The listing builds one solid part. Answer for the finished solid, in the listing's coordinates (mm). A direction names the side the tool comes from. Coordinates: 2 decimals unless noted, no trailing zeros. Order: outer loops, then holes, each group sorted by start corner. A loop starts at its lowest first (then second) coordinate and runs counter-clockwise, first axis right, second up. Notation, with made-up numbers: M 74,-26 L 93,-26 A25 ccw 93,11 Z; hole C -16,89.5 d11. An arc over 180 degrees is marked long. One line per item, written item: value. Start each with the question number.
Q1. The part is cut by section C-C on z = 73. Give the vertices of the cut face in (x, y).
Q2. The part is cut by section A-A on y = -196. Give the vertices of the cut face in (x, z).
Q3. Straight lines are drawn through the part: line 1 along Y through (x, z) = (38.5, 49); line 2 along Z through (x, y) = (166.5, -106.5); line 3 along Z through (x, y) = (140, -156). For each, find the intervals that lie inside material, in ascending order. Write a range as [from, to].
Q4. The part is cut by section B-B on x = 130. Give the vertices of the cut face in (y, z), then the cut area to 3 significant figures.
Q5. For faces 1 (the flat face through (160, 0, 65)), 2 (the cylindrical face through (68.872, -33.32, 32.944)), determine the directions among +Z, -Z, +X, -X, +Y, -Y from which every point of the face is accessible in a straight line to the end or side of a thin tool.
Q6. The part is cut by section D-D on x = 160.5. Give the vertices of the cut face in (y, z), then the cut area to 3 significant figures.
Q7. Each of these flat-tipped pins is pushed along its axis until it touches: pin 1 Ø2 at (y, z) = (-89, 57) entering from -X; pin 2 Ø3 at (x, y) = (119.5, -97) entering from -Z; pin 3 Ø6 at (x, z) = (138, 78) entering from -Y; pin 4 Ø2 at (x, y) = (120, -38.5) entering from +Z. Where does it stop, or does it pass through?
```python
from build123d import *

# Parameters (mm, degrees)
F1_R     = 17.586867
F2_DEPTH = 139.7
F3_DEPTH = 228.346


with BuildPart() as f2:
    # F1 (on Right) → F2 (new body)
    with BuildSketch(Plane.YZ):
        with Locations((-41.434839, 48.546314)):
            Circle(F1_R)
    extrude(amount=F2_DEPTH)

    # F0 (on Front) → F3 (join)
    with BuildSketch(Plane.XZ):
        Polygon((173.909366, 88.873066), (119.005956, 67.850798), (143.216059, 49.334605), (173.909366, 49.334605), (187.112732, 54.390115), align=None)
    extrude(amount=F3_DEPTH)


solid = f2.part
```
Output:
1. outline: M 132.45,-228.35 L 179.99,-228.35 L 179.99,0 L 132.45,0 Z
2. outline: M 119.01,67.85 L 143.22,49.33 L 173.91,49.33 L 187.11,54.39 L 173.91,88.87 Z
3. line 1: y = [-59.02, -23.85]
3. line 2: z = [49.33, 86.04]
3. line 3: z = [51.79, 75.89]
4. outline: M -228.35,59.44 L -55.24,59.44 A17.59 ccw long -27.63,59.44 L 0,59.44 L 0,72.06 L -228.35,72.06 Z
4. area: 3,720 mm^2
5. face 1: +Z, -Z, +X, -X, +Y
5. face 2: -X
6. outline: M -228.35,49.33 L 0,49.33 L 0,83.74 L -228.35,83.74 Z
6. area: 7,860 mm^2
7. pin 1: stops at x = 131.89
7. pin 2: stops at z = 66.33
7. pin 3: stops at y = -228.35
7. pin 4: stops at z = 68.61
